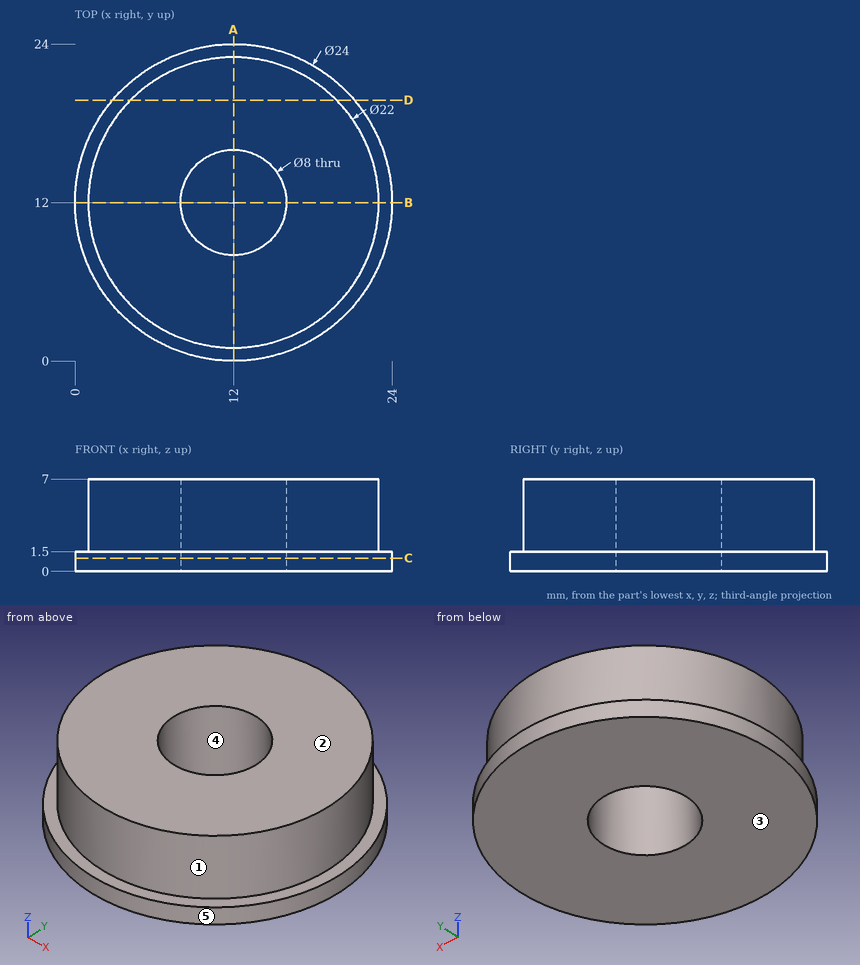
Study the drawing (mm; zero at the part's minimum x, y, z) and answer. A direction names the side the tool comes from. Give positions to 0.01 mm unless a question says otherwise; leave off trailing zeros. Order: outer loops, then holes, each group sorted by start corner. A loop starts at its lowest first (then second) coordinate and runs counter-clockwise, first axis right, second up.
1) For the marked faces 1 and 2, determine the directions among +Z, -Z, +X, -X, +Y, -Y from which every point of the face is accessible in a straight line to the end or side of a thin tool.
Reported:
face 1: +Z
face 2: +Z, +X, -X, +Y, -Y
2) Find section A-A on x = 12. Write down the section's boundary in (y, z).
Reported:
outline: (0, 0) - (8, 0) - (8, 7) - (1, 7) - (1, 1.5) - (0, 1.5) - close; (16, 0) - (24, 0) - (24, 1.5) - (23, 1.5) - (23, 7) - (16, 7) - close
3) Find section D-D on y = 19.75. Write down the section's boundary in (x, z), then the cut area to 3 significant figures.
Reported:
outline: (2.84, 0) - (21.16, 0) - (21.16, 1.5) - (19.81, 1.5) - (19.81, 7) - (4.19, 7) - (4.19, 1.5) - (2.84, 1.5) - close
area: 113 mm2
4) Find section C-C on z = 1. Write down the section's boundary in (x, y), then the cut area to 3 significant figures.
Reported:
outline: circle Ø24 at (12, 12); hole circle Ø8 at (12, 12)
area: 402 mm2
5) Determine the mould class of the marked faces 3, 4 and 5 for opening direction Y: pulls with the +Y half, pulls with the -Y half, needs draft (parallel to the pull), parting line crosses it, or undercut.
Reported:
face 3: needs draft
face 4: undercut
face 5: parting line crosses it
6) Consider line 1 along Y through (x, z) = (12, 1.75); line 2 along Y through (x, z) = (9.25, 6.5); line 3 along X through (y, z) = (14.5, 0.75). Determine where each line is inside the solid, lowest interval first.
Reported:
line 1: y = 1 to 8, 16 to 23
line 2: y = 1.35 to 9.1, 14.9 to 22.65
line 3: x = 0.26 to 8.88, 15.12 to 23.74
7) Given P1, Ø1.5, axis at x = 6.5, z = 3, coming from the -Y side; P2, Ø1.5, axis at x = 12.5, y = 9.5, coming from the -Z side; P3, Ø4, axis at y = 6, z = 5.5, coming from the +X side, each flat-ended and moving along its own axis, determine where each tip first touches the part or whether it passes through.
Reported:
P1: stops at y = 2.08
P2: passes through
P3: stops at x = 22.25
